Work out the finished part from the listing and answer in its coordinate system (mm). A direction names the side the tool comes from. Round coordinates to 2 decimals unless told otherwise and drop trailing zeros. Order: outer loops, then holes, each group sorted by start corner. A loop starts at its lowest first (then second) coordinate and runs counter-clockwise, first axis right, second up. Notation, with made-up numbers: (-11, -40) - (29, -40) arc R27 cw to (29, -21) - close; hole circle Ø1 at (-5.5, 75.5). An arc over 180 degrees is marked (long way). Use one line per item in the form item = value. Start each with the question number.
Q1. For a pull along X with two mould halves and no side action, classify faces 3 (the cylindrical face through (5.506, 11.988, -24.796)), 4 (the flat face through (0, 31.75, 0)), 5 (the cylindrical face through (3.85, 2.95, 17.36)), 6 (the cylindrical face through (5.506, -7.56, -24.796)) as +X half, -X half, draft (parallel to the pull), parting line (faces both ways), or undercut.
Q2. Find the intervals of material crossed by line 1 (Z direction, x = 0, y = 7); line 2 (Y direction, x = -21.5, z = -12); line 3 (X direction, y = 8, z = 23), in increasing order. Write a range as [from, to].
Q3. Given P1, Ø10, axis at x = 19.5, y = 5, coming from the +Z side; P2, Ø6, axis at y = 1.5, z = -13, coming from the +X side; P3, Ø12, axis at x = -14.5, y = 26.5, coming from the -Z side, each flat-ended and moving along its own axis, determine where each tip first touches the part or whether it passes through.
Q4. The part is cut by section A-A on y = 15.5. Determine the outline of the cut face in (x, z), plus the area to 3 significant figures.
Q5. Which of the six approach directions +Z, -Z, +X, -X, +Y, -Y give full straight-line access (tool end or side, diameter ignored) to faces 1 (the cylindrical face through (-31.406, 5.593, -0.145)), 2 (the cylindrical face through (6.607, 9.392, 29.755))?
Q6. The part is cut by section B-B on y = 8.89. Determine the outline of the cut face in (x, z), plus the area to 3 significant figures.
Q7. The part is cut by section C-C on y = 21.5. Determine the outline of the cut face in (x, z), plus the area to 3 significant figures.
Autodesk Inventor part; units mm, degrees
ref_plane "Work Plane4" through (-32.48, 0, 0) normal (1, 0, 0) x (0, 1, 0)
ref_plane "Work Plane5" through (30.48, 0, 0) normal (1, 0, 0) x (0, 1, 0)
ref_plane "XZ Plane" through (0, 0, 0) normal (0, 1, 0) x (-1, 0, 0)
sketch "Sketch1" plane through (0, 0, 0) normal (0, 1, 0) x (-1, 0, 0)
  circle A0 centre (0, 0) radius 30.48
  circle A1 centre (0, 0) radius 32.48
  dimension "d0" = 60.96
  dimension "d2" = 2
extrude "Extrusion1" add sketch "Sketch1" along normal blind 19.05
sketch "Sketch2" plane through (0, 19.05, 0) normal (0, 1, 0) x (1, 0, 0)
  circle A0 centre (0, 0) radius 32.48
  circle A1 centre (0, 0) radius 32.48
extrude "Extrusion2" add sketch "Sketch2" along normal blind 12.7
fillet "Fillet1" radius 6.35 1 edges at (-32.48, 31.75, 0)
sketch "Sketch10" plane through (0, 0, 0) normal (0, 0, 1) x (1, 0, 0)
  line L0 (-17.78, 19.05) -> (-17.78, -12.7)
  line L1 (-17.78, -12.7) -> (-25.4, -12.7)
  line L2 (-25.4, -12.7) -> (-25.4, 19.05)
  line L3 (-17.78, 19.05) -> (-25.4, 19.05)
  line L4 (-26.13, 31.75) -> (26.13, 31.75)
  line L5 (0, 31.75) -> (0, 0)
  line L6 (32.48, 0) -> (-32.48, 0)
  line L7 (-30.48, 0) -> (-30.48, 19.05)
  line L8 (-17.78, -12.7) -> (-25.4, -8.3006)
  line L9 (-30.48, 19.05) -> (30.48, 19.05)
  point P0 (-30.48, 0)
  point P1 (-25.4, 19.05)
  dimension "d29" = 7.62
  dimension "d33" = 30
  dimension "d42" = 25.4
  dimension "d89" = 31.75
revolve "Revolution2" add sketch "Sketch10" angle 360 about axis through (0, 31.75, 0) along (0, -1, 0) contours L0 L6 L2 L3 | L0 L8 L2 L6
sketch "Sketch11" plane through (0, 0, 0) normal (0, 0, 1) x (1, 0, 0)
  line L0 (25.4, -7.0306) -> (25.4, 25.4)
  circle A0 centre (26.3462, -3.81) radius 3.175
  circle A1 centre (26.3462, 2.54) radius 2.3813
  line L1 (0, -11.43) -> (0, 31.75)
  line L2 (-26.13, 31.75) -> (26.13, 31.75)
  line L3 (26.3462, 2.54) -> (26.3462, -3.81)
  line L4 (30.48, 19.05) -> (30.48, 0)
  line L5 (30.48, 0) -> (29.972, 19.05)
  line L6 (29.972, 19.05) -> (29.972, 0)
  line L7 (-25.4, -5.08) -> (25.4, -5.08)
  line L8 (-17.78, -12.7) -> (17.78, -12.7)
  point P0 (0, 0)
  point P1 (25.4, -8.3006)
  point P2 (27.772, -0.6806)
  point P3 (17.78, -12.7)
  dimension "d36" = 6.35
  dimension "d37" = 4.7625
  dimension "d38" = 6.35
  dimension "d43" = 26.3462
  dimension "d91" = 8.89
revolve "Revolution3" cut sketch "Sketch11" angle 360 about axis through (0, -11.43, 0) along (0, 1, 0) contours A0 L7 L0 | L0 A0 | L7 A0 L0 | A1 L0 | L0 A1
ref_plane "Work Plane4" through (-32.48, 0, 0) normal (1, 0, 0) x (0, 1, 0)
sketch "Sketch24" plane through (-32.48, 0, 0) normal (1, 0, 0) x (0, 1, 0)
  circle A0 centre (8.89, 0) radius 3.3
  line L0 (0, -32.48) -> (0, 32.48)
  line L1 (31.75, 5) -> (31.75, -5)
  line L2 (31.75, 0) -> (0, 0) construction
  line L3 (-0.7793, -25.4) -> (-0.7793, 25.4)
  dimension "d106" = 6.6
  dimension "d107" = 8.89
  dimension "d108" = 0
extrude "Extrusion16" cut sketch "Sketch24" along normal up to surface
ref_plane "Work Plane5" through (30.48, 0, 0) normal (1, 0, 0) x (0, 1, 0)
properties part number "Water_Sensor_Cap_3DPrint"
Found:
q1.face_3 = undercut
q1.face_4 = draft
q1.face_5 = undercut
q1.face_6 = parting line
q2.line_1 = [-32.48, -30.48], [-25.4, -17.78], [17.78, 25.4], [30.48, 32.48]
q2.line_2 = [-8.75, -6.48], [-1.14, 0.9], [4.18, 31.75]
q2.line_3 = [-22.93, -20], [-10.78, 10.78], [20, 22.93]
q3.P1 = 29.06
q3.P2 = 30.9
q3.P3 = -31.33
q4.outline = circle Ø64.96 at (0, 0); circle Ø50.8 at (0, 0); hole circle Ø60.96 at (0, 0); hole circle Ø35.56 at (0, 0)
q4.area = 1,430 mm²
q5.face_1 = -X
q5.face_2 = -Y
q6.outline = (-32.31, -3.3) arc R32.48 ccw (long way) to (-32.31, 3.3) - (-30.3, 3.3) arc R30.48 cw (long way) to (-30.3, -3.3) - close; circle Ø50.8 at (0, 0); hole circle Ø35.56 at (0, 0)
q6.area = 1,420 mm²
q7.outline = circle Ø64.96 at (0, 0)
q7.area = 3,310 mm²
